Autodesk Inventor part; units mm, degrees
ref_plane "YZ Plane" through (0, 0, 0) normal (1, 0, 0) x (0, 1, 0)
ref_plane "XZ Plane" through (0, 0, 0) normal (0, 1, 0) x (-1, 0, 0)
ref_plane "XY Plane" through (0, 0, 0) normal (0, 0, 1) x (1, 0, 0)
sketch "Sketch1" plane through (0, 0, 0) normal (1, 0, 0) x (0, 1, 0)
  line L0 (0, 0) -> (10.9, 0)
  line L1 (10.9, 0) -> (10.9, -85.6)
  line L2 (10.9, -85.6) -> (0, -85.6)
  line L3 (0, -85.6) -> (0, -59)
  line L4 (-9.75, -85.6) -> (-9.75, -65.3)
  line L5 (-9.75, -65.3) -> (-9.75, -10.8)
  line L6 (-9.75, -65.3) -> (0, -59)
  line L7 (0, 0) -> (0, -17)
  line L8 (0, -17) -> (-9.75, -10.8)
  dimension "d1" = 85.6
  dimension "d2" = 26.6
  dimension "d5" = 20.3
  dimension "d6" = 54.5
  dimension "d7" = 17
extrude "Extrusion1" add sketch "Sketch1" against normal blind 165.2
sketch "Sketch2" plane through (0, 10.9, 0) normal (0, 1, 0) x (1, 0, 0)
  point P0 (0, 0)
sketch "Sketch3" plane through (0, 10.9, 0) normal (0, 1, 0) x (1, 0, 0)
  line L0 (0, 0) -> (0, 85.6)
  line L1 (0, 42.8) -> (-14, 42.8)
  line L2 (-14, 42.8) -> (-82.3, 42.8)
  circle A0 centre (-82.3, 42.8) radius 68.3
  dimension "d10" = 14
  dimension "d11" = 68.3
extrude "Extrusion2" add sketch "Sketch3" along normal blind 11.5
sketch "Sketch4" plane through (-82.3, 22.4, -42.8) normal (0, 1, 0) x (1, 0, 0)
  circle A0 centre (0, 0) radius 9.15
  point P0 (82.3, -42.8)
  dimension "d14" = 18.3
extrude "Extrusion3" cut sketch "Sketch4" against normal blind 73.75
sketch "Sketch5" plane through (-82.3, 22.4, -42.8) normal (0, 1, 0) x (1, 0, 0)
  circle A0 centre (0, 0) radius 68.3
  line L0 (0, 68.3) -> (0, 62.3)
  line L1 (0, -68.3) -> (0, -62.3)
  line L2 (0, 62.3) -> (0, 56.9)
  circle A1 centre (0, 56.9) radius 5.4
  line L3 (0, -62.3) -> (0, -56.9)
  line L4 (82.3, -32) -> (-82.9, -32)
  circle A2 centre (0, -56.9) radius 5.4
  point P0 (82.3, -42.8)
  dimension "d17" = 6
  dimension "d18" = 6
  dimension "d19" = 5.4
  dimension "d20" = 5.4
extrude "Extrusion4" cut sketch "Sketch5" against normal blind 73.75 contours A1 | A2
sketch "Sketch6" plane through (-82.3, 22.4, -42.8) normal (0, 1, 0) x (1, 0, 0)
  point P0 (82.3, -42.8)
sketch "Sketch7" plane through (-82.3, 22.4, -42.8) normal (0, 1, 0) x (1, 0, 0)
  circle A0 centre (0, 0) radius 68.3
  line L0 (68.3, 0) -> (61.4, 0)
  line L1 (61.4, 0) -> (50.6, 0)
  circle A1 centre (50.6, 0) radius 10.8
  point P0 (82.3, -42.8)
  dimension "d23" = 6.9
  dimension "d24" = 10.8
extrude "Extrusion5" cut sketch "Sketch7" against normal blind 6 contours A1
sketch "Sketch8" plane through (-31.7, 16.4, -42.8) normal (0, 1, 0) x (1, 0, 0)
  circle A0 centre (0, 0) radius 3.1
  point P0 (31.7, -42.8)
  dimension "d27" = 6.2
extrude "Extrusion6" cut sketch "Sketch8" against normal blind 22.8
properties part number "Top Part Tool bit"
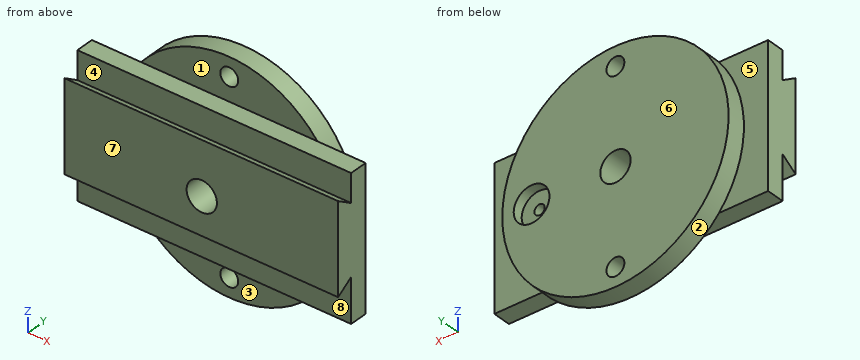
Verification items for the finished model (mm, model axes). Face numbers are marked on the shaded views. A direction names the side the tool comes from. Round coordinates to 2 decimals unless told otherwise and drop trailing zeros. Write each loop counter-clockwise with the first axis right and the second up, starting at its lowest first coordinate (ties: lowest second). Pieces come first, ordered by that corner, then holes.
(1) Section check D-D (z = -76.5). Enter the section's corners in (x, y).
Returned:
outline: (-165.2, 0) - (0, 0) - (0, 10.9) - (-22.89, 10.9) - (-22.89, 22.4) - (-141.71, 22.4) - (-141.71, 10.9) - (-165.2, 10.9) - close
(2) Section check A-A (z = -42.8). Enter the section's corners in (x, y).
Returned:
outline: (-165.2, -9.75) - (-91.45, -9.75) - (-91.45, 22.4) - (-150.6, 22.4) - (-150.6, 10.9) - (-165.2, 10.9) - close; (-73.15, -9.75) - (0, -9.75) - (0, 10.9) - (-14, 10.9) - (-14, 22.4) - (-20.9, 22.4) - (-20.9, 16.4) - (-28.6, 16.4) - (-28.6, -6.4) - (-34.8, -6.4) - (-34.8, 16.4) - (-42.5, 16.4) - (-42.5, 22.4) - (-73.15, 22.4) - close
(3) Material ranges on line 1 (X direction, y = 6.75, z = -42.8); line 2 (Z direction, x = -82.3, y = 17.25); line 3 (X direction, y = 18, z = -42), recorded low to high.
Returned:
line 1: x = -165.2 to -91.45, -73.15 to -34.8, -28.6 to 0
line 2: z = -111.1 to -105.1, -94.3 to -51.95, -33.65 to 8.7, 19.5 to 25.5
line 3: x = -150.6 to -91.41, -73.19 to -42.47, -20.93 to -14
(4) Depth check by flat-ended pin: pin 1 Ø9.5 at (x, z) = (-82.3, -99.7) entering from +Y; pin 2 Ø1.5 at (x, y) = (-26.5, 5.5) entering from -Z; pin 3 Ø7.5 at (x, z) = (-60, -103) entering from -Y; pin 4 Ø1.5 at (x, y) = (-86.5, 17.5) entering from +Z. Enter the tip coordinate at first touch or a pass-through.
Returned:
pin 1: passes through
pin 2: stops at z = -85.6
pin 3: stops at y = 10.9
pin 4: stops at z = 25.41
(5) Access from +Z, -Z, +X, -X, +Y, -Y to the whole of each face (thin tool, end or side, straight path). Record for the marked faces 1, 2, 3, 4 and 5.
Returned:
face 1: +Z, +X, -X, -Y
face 2: +Y
face 3: -Z, +X, -X, -Y
face 4: +Z, +X, -X
face 5: -X, +Y
(6) Mould release check, pull along Y, two halves, no side actions. Record for the marked faces 6, 7 and 8: pulls with the +Y half, pulls with the -Y half, needs draft (parallel to the pull), parting line crosses it, or undercut.
Returned:
face 6: pulls with the +Y half
face 7: pulls with the -Y half
face 8: undercut
(7) Section check B-B (y = 2). Enter the section's corners in (x, z).
Returned:
outline: (-165.2, -85.6) - (0, -85.6) - (0, 0) - (-165.2, 0) - close; hole circle Ø18.3 at (-82.3, -42.8); hole circle Ø6.2 at (-31.7, -42.8)
(8) Section check C-C (x = -69). Enter the section's corners in (y, z).
Returned:
outline: (-9.75, -65.3) - (0, -59) - (0, -85.6) - (10.9, -85.6) - (10.9, -109.79) - (22.4, -109.79) - (22.4, 24.19) - (10.9, 24.19) - (10.9, 0) - (0, 0) - (0, -17) - (-9.75, -10.8) - close
